Verification items for the finished model (mm, model axes). A direction names the side the tool comes from. Give positions to 0.01 mm unless a question says otherwise; leave off trailing zeros.
(1) Gauge pin test, flat ends, axial feed: pin 1 (21 mm diameter, centred on x = 51.5, y = 30.5, fed in from -Z); pin 2 (10 mm diameter, centred on x = -4, y = 78, fed in from -Z); pin 3 (2 mm diameter, centred on x = -39.5, y = 26.5, fed in from +Z). Record the tip position at first contact, or that the pin passes through.
(2) Scan lines: L1, parallel to Y at x = 0, z = 2; L2, parallel to Y at x = 0, z = 8.2; L3, parallel to X at y = -8.5, z = -42. Record each from-to range of solid material in increasing order.
(3) Mould release check, pull along Z, two halves, no side actions. Record for faces 4 (the face through (-108, 0, -86.732)), 5 (the face through (42, 42, 1)), 6 (the face through (47.69, 15.02, 7.46)): pulls with the +Z half, pulls with the -Z half, needs draft (parallel to the pull), parting line crosses it, or undercut.
(4) Access from +Z, -Z, +X, -X, +Y, -Y to the whole of each face (thin tool, end or side, straight path). Record for faces 1 (the face through (-41.591, -38.056, 1.208)), 2 (the face through (0, 108, -86.732)), 3 (the face through (-55.55, -42.594, 4.93)).
(5) Sectioned sample at A-A on z = -33.5. Count the separate pieces of the cut face and the enclosed holes in it, plus the area to 3 significant figures.
```python
from build123d import *

# Parameters (mm, degrees)
SKETCH1_R           = 70
SKETCH1_R_2         = 50
BOSS_EXTRUDE1_DEPTH = 10
SKETCH1_6_R         = 50
SKETCH1_6_R_2       = 45
BOSS_EXTRUDE3_DEPTH = 5
SKETCH2_R           = 12.5
CIRPATTERN2_COUNT   = 4
CUT_EXTRUDE5_DEPTH  = 2
CUT_EXTRUDE8_START  = -1
CUT_EXTRUDE8_DEPTH  = 1
CIRPATTERN4_COUNT   = 4


with BuildPart() as part:
    # Sketch1 → Boss-Extrude1 (new body)
    with BuildSketch(Plane.XY):
        Circle(SKETCH1_R)
        Circle(SKETCH1_R_2, mode=Mode.SUBTRACT)
    extrude(amount=BOSS_EXTRUDE1_DEPTH)

    # Sketch1_6 → Boss-Extrude3 (add)
    with BuildSketch(Plane.XY):
        Circle(SKETCH1_6_R)
        Circle(SKETCH1_6_R_2, mode=Mode.SUBTRACT)
    extrude(amount=BOSS_EXTRUDE3_DEPTH)

    # Sweep1: sweep along a path in Sketch3
    with BuildLine(Plane(origin=(0, 0, 0), x_dir=(0, 0, -1), z_dir=(1, 0, 0))) as sweep1_path:
        Line((0, -57.5), (86.731949901, -107.982962913))
    # Sketch2 → Sweep1 (sweep)
    with BuildSketch(Plane(origin=(0, 0, 0), x_dir=(-1, 0, 0), z_dir=(0, 0, -1))):
        with Locations((0, -57.5)):
            Circle(SKETCH2_R)
    sweep1 = sweep(path=sweep1_path.line)

    # CirPattern2: Sweep1 ×4 about axis
    cirpattern2_axis = Axis((0, 0, 10), (0, 0, -1))
    for i in range(1, CIRPATTERN2_COUNT):
        add(sweep1.rotate(cirpattern2_axis, i * 360 / CIRPATTERN2_COUNT))

    # Sketch8 → Cut-Extrude5 (cut)
    with BuildSketch(Plane(origin=(0, 0, 0), x_dir=(-1, 0, 0), z_dir=(0, 0, -1))):
        Polygon((-38.890872965, 42.426406871), (-35.355339059, 38.890872965), (-38.890872965, 35.355339059), (-42.426406871, 38.890872965), align=None)
    cut_extrude5 = extrude(amount=-CUT_EXTRUDE5_DEPTH, mode=Mode.SUBTRACT)

    # Sketch8_6 → Cut-Extrude8 (cut)
    with BuildSketch(Plane(origin=(0, 0, 0), x_dir=(-1, 0, 0), z_dir=(0, 0, -1)).offset(CUT_EXTRUDE8_START)):
        Polygon((-42.426406871, 38.890872965), (-45.961940777, 42.426406871), (-42.426406871, 45.961940777), (-38.890872965, 42.426406871), align=None)
    cut_extrude8 = extrude(amount=-CUT_EXTRUDE8_DEPTH, mode=Mode.SUBTRACT)

    # CirPattern4: Cut-Extrude5, Cut-Extrude8 ×4 about axis
    cirpattern4_axis = Axis((0, 0, 0), (0, 0, 1))
    for i in range(1, CIRPATTERN4_COUNT):
        add(cut_extrude5.rotate(cirpattern4_axis, i * 360 / CIRPATTERN4_COUNT), mode=Mode.SUBTRACT)
        add(cut_extrude8.rotate(cirpattern4_axis, i * 360 / CIRPATTERN4_COUNT), mode=Mode.SUBTRACT)


solid = part.part
```
Ans:
1. pin 1: stops at z = 0
1. pin 2: stops at z = -64.49
1. pin 3: stops at z = 5
2. L1: y = -70 to -45, 45 to 70
2. L2: y = -70 to -50, 50 to 70
2. L3: x = -91.11 to -72.78, 72.78 to 91.11
3. face 4: pulls with the -Z half
3. face 5: undercut
3. face 6: needs draft
4. face 1: none
4. face 2: -Z, +X, -X, +Y, -Y
4. face 3: +Z
5. separate pieces: 4
5. enclosed holes: 0
5. area: 1,960 mm2
